Here's how the part is built. I have some questions about the finished solid (model axes, mm). Give positions to 0.01 mm unless a question says otherwise; leave off trailing zeros. Loops run counter-clockwise (first coordinate to the right, second up) from the corner with the lowest first, then second, coordinate; pieces in that order, holes last.
Q1. Thinking about a two-plate mould opening in X: for faces 1 (the face through (0, 0, 145)), 2 (the face through (0, 1.4, 145)), which applies, pulls with the +X half, pulls with the -X half, needs draft (parallel to the pull), parting line crosses it, or undercut?
Q2. Suppose I cut it at A-A (y = 4.5). List the corners of the cut face in (x, z) for me.
Q3. Suppose I cut it at C-C (x = 8.5). List the corners of the cut face in (y, z) for me, and give its area (3 significant figures).
Q4. I'm going to push flat-ended pins straight in: P1, Ø0.6, axis at x = -17, z = 179, coming from the -Y side; P2, Ø1.6, axis at y = 4.5, z = 183.5, coming from the +X side; P3, Ø2.5, axis at y = 3.5, z = 125, coming from the -X side. Where does each tip first touch, or does it pass through?
Q5. Suppose I cut it at B-B (z = 213). List the corners of the cut face in (x, y) for me, and give its area (3 significant figures).
Q6. I need wall thicknesses on probe 1 along X at (y, z) = (5, 93); probe 2 along Y at (x, z) = (0, 258); probe 3 along X at (y, z) = (6.25, 122.5). Which ranges of each line are inside material? Lowest first, please.
```python
from build123d import *

# Parameters (mm, degrees)
BOSS_EXTRUDE1_DEPTH = 295


with BuildPart() as part:
    # Sketch1 → Boss-Extrude1 (new body)
    with BuildSketch(Plane.XY):
        with BuildLine():
            Line((-15.5, 0), (15.5, 0))
            Line((15.5, 0), (13.5, 2.6))
            Line((13.5, 2.6), (13.5, 5.8))
            Line((13.5, 5.8), (15.3, 6.92))
            Line((15.3, 6.92), (17.4, 6.92))
            Line((17.4, 6.92), (17.4, 7.82))
            Line((17.4, 7.82), (14.6, 7.82))
            ThreePointArc((14.6, 7.82), (13.185786438, 7.234213562), (12.6, 5.82))
            Line((12.6, 5.82), (12.6, 1.4))
            Line((12.6, 1.4), (-12.6, 1.4))
            Line((-12.6, 1.4), (-12.6, 5.82))
            ThreePointArc((-12.6, 5.82), (-13.185786438, 7.234213562), (-14.6, 7.82))
            Line((-14.6, 7.82), (-17.4, 7.82))
            Line((-17.4, 7.82), (-17.4, 6.92))
            Line((-17.4, 6.92), (-15.3, 6.92))
            Line((-15.3, 6.92), (-13.5, 5.8))
            Line((-13.5, 5.8), (-13.5, 2.6))
            Line((-13.5, 2.6), (-15.5, 0))
        make_face()
    extrude(amount=BOSS_EXTRUDE1_DEPTH)


solid = part.part
```
Solutions:
1. face 1: needs draft
1. face 2: undercut
2. outline: (-13.5, 0) - (-12.6, 0) - (-12.6, 295) - (-13.5, 295) - close; (12.6, 0) - (13.5, 0) - (13.5, 295) - (12.6, 295) - close
3. outline: (0, 0) - (1.4, 0) - (1.4, 295) - (0, 295) - close
3. area: 413 mm2
4. P1: stops at y = 6.92
4. P2: stops at x = 13.5
4. P3: stops at x = -13.77
5. outline: (-17.4, 6.92) - (-15.3, 6.92) - (-13.5, 5.8) - (-13.5, 2.6) - (-15.5, 0) - (15.5, 0) - (13.5, 2.6) - (13.5, 5.8) - (15.3, 6.92) - (17.4, 6.92) - (17.4, 7.82) - (14.6, 7.82) arc R2 ccw to (12.6, 5.82) - (12.6, 1.4) - (-12.6, 1.4) - (-12.6, 5.82) arc R2 ccw to (-14.6, 7.82) - (-17.4, 7.82) - close
5. area: 61.9 mm2
6. probe 1: x = -13.5 to -12.6, 12.6 to 13.5
6. probe 2: y = 0 to 1.4
6. probe 3: x = -14.22 to -12.65, 12.65 to 14.22
